Geometry check sheet. Reference: the model listing, model coordinates, mm. A direction names the side the tool comes from. Give positions to 0.01 mm unless a question says otherwise; leave off trailing zeros. Write each loop counter-clockwise with the first axis right and the second up, starting at its lowest first coordinate (ties: lowest second). Pieces come first, ordered by that corner, then holes. Notation, with made-up numbers: (36, 1.5) - (80, 1.5) arc R17 cw to (80, 13.5) - close; hole circle Ø6 at (-12.75, 73.5). An arc over 180 degrees is marked (long way). Write item = value, one per line. Start each with the question number.
(1) Depth check by flat-ended pin: pin 1 Ø1.5 at (x, y) = (-13, -8) entering from +Z; pin 2 Ø1.2 at (x, y) = (21, 17) entering from +Z; pin 3 Ø3 at (x, y) = (22.75, -17.5) entering from -Z. Enter the tip coordinate at first touch or a pass-through.
(2) Section check D-D, the plane y = 17.5. Enter the section's corners in (x, z).
(3) Section check A-A, the plane y = 0. Enter the section's corners in (x, z), plus the area to 3 significant figures.
(4) Section check B-B, the plane x = 16. Enter the section's corners in (y, z).
(5) Draft check along X on faces 4 (the flat face through (-23, -17, 6)), 5 (the flat face through (-21, -18, 1)), 6 (the flat face through (-24.2, 11.2, 18)), 7 (the flat face through (20, 17, 5)). Enter one of: pulls with the +X half, pulls with the -X half, needs draft (parallel to the pull), parting line crosses it, or undercut.
(6) Thickness scan on L1, parallel to Y at x = 22.75, z = 4.35; L2, parallel to X at y = -23, z = 17.25; L3, parallel to X at y = -17.5, z = 6.75. Record the ranges inside material, lowest first.
(7) Access from +Z, -Z, +X, -X, +Y, -Y to the whole of each face (thin tool, end or side, straight path). Record for faces 1 (the flat face through (-23, 18, 6)), 2 (the flat face through (-22, 18, 7)), 3 (the flat face through (-23, 15.5, 1)).
```python
from build123d import *

# Parameters (mm, degrees)
SKICA1_W                  = 50
SKICA1_H                  = 50
P_IDAT_VYSUNUT_M2_DEPTH   = 3
SKICA5_W                  = 50
SKICA5_H                  = 5
ODEBRAT_VYSUNUT_M3_DEPTH  = 1
P_IDAT_VYSUNUT_M9_DEPTH   = 15
SKICA17_R                 = 2
ODEBRAT_VYSUNUT_M8_DEPTH  = 4
SKICA18_W                 = 5
SKICA18_H                 = 5
P_IDAT_VYSUNUT_M10_DEPTH  = 7
SKICA19_W                 = 4
SKICA19_H                 = 4
ODEBRAT_VYSUNUT_M9_DEPTH  = 3
SKICA20_R                 = 1.25
ODEBRAT_VYSUNUT_M10_DEPTH = 3


with BuildPart() as part:
    # Skica1 → Přidat vysunutím2 (new body)
    with BuildSketch(Plane.XY):
        Rectangle(SKICA1_W, SKICA1_H)
    extrude(amount=P_IDAT_VYSUNUT_M2_DEPTH)

    # Skica5 → Odebrat vysunutím3 (cut)
    with BuildSketch(Plane(origin=(0, 0, 0), x_dir=(-1, 0, 0), z_dir=(0, 0, -1))):
        Rectangle(SKICA5_W, SKICA5_H)
    extrude(amount=-ODEBRAT_VYSUNUT_M3_DEPTH, mode=Mode.SUBTRACT)

    # Skica14 → Přidat vysunutím9 (add)
    with BuildSketch(Plane.XY.offset(3)):
        Polygon((25, 25), (-25, 25), (-25, -25), (-24, -25), (-24, 24), (24, 24), (24, -25), (25, -25), align=None)
    extrude(amount=P_IDAT_VYSUNUT_M9_DEPTH)

    # Skica17 → Odebrat vysunutím8 (cut)
    with BuildSketch(Plane(origin=(0, 0, 1), x_dir=(-1, 0, 0), z_dir=(0, 0, -1))):
        with Locations((-16, 0)):
            Circle(SKICA17_R)
        with Locations((16, 0)):
            Circle(SKICA17_R)
    extrude(amount=-ODEBRAT_VYSUNUT_M8_DEPTH, mode=Mode.SUBTRACT)

    # Skica18 → Přidat vysunutím10 (add)
    with BuildSketch(Plane(origin=(0, 0, 0), x_dir=(-1, 0, 0), z_dir=(0, 0, -1))):
        with Locations((-22.5, 17.5)):
            Rectangle(SKICA18_W, SKICA18_H)
        with Locations((-22.5, -17.5)):
            Rectangle(SKICA18_W, SKICA18_H)
        with Locations((22.5, -17.5)):
            Rectangle(SKICA18_W, SKICA18_H)
        with Locations((22.5, 17.5)):
            Rectangle(SKICA18_W, SKICA18_H)
    extrude(amount=-P_IDAT_VYSUNUT_M10_DEPTH)

    # Skica19 → Odebrat vysunutím9 (cut)
    with BuildSketch(Plane(origin=(0, 0, 0), x_dir=(-1, 0, 0), z_dir=(0, 0, -1))):
        with Locations((-23, 17.5)):
            Rectangle(SKICA19_W, SKICA19_H)
        with Locations((-23, -17.5)):
            Rectangle(SKICA19_W, SKICA19_H)
        with Locations((23, -17.5)):
            Rectangle(SKICA19_W, SKICA19_H)
        with Locations((23, 17.5)):
            Rectangle(SKICA19_W, SKICA19_H)
    extrude(amount=-ODEBRAT_VYSUNUT_M9_DEPTH, mode=Mode.SUBTRACT)

    # Skica20 → Odebrat vysunutím10 (cut)
    with BuildSketch(Plane(origin=(0, 0, 3), x_dir=(-1, 0, 0), z_dir=(0, 0, -1))):
        with Locations((-22.75, 17.5)):
            Circle(SKICA20_R)
        with Locations((22.75, 17.5)):
            Circle(SKICA20_R)
        with Locations((22.75, -17.5)):
            Circle(SKICA20_R)
        with Locations((-22.75, -17.5)):
            Circle(SKICA20_R)
    extrude(amount=-ODEBRAT_VYSUNUT_M10_DEPTH, mode=Mode.SUBTRACT)


solid = part.part
```
Model answer:
q1.pin_1 = 3
q1.pin_2 = 7
q1.pin_3 = 3
q2.outline = (-25, 3) - (-24, 3) - (-24, 6) - (-21.5, 6) - (-21.5, 3) - (-21, 3) - (-21, 0) - (21, 0) - (21, 3) - (21.5, 3) - (21.5, 6) - (24, 6) - (24, 3) - (25, 3) - (25, 18) - (24, 18) - (24, 7) - (20, 7) - (20, 3) - (-20, 3) - (-20, 7) - (-24, 7) - (-24, 18) - (-25, 18) - close
q3.outline = (-25, 1) - (-18, 1) - (-18, 3) - (-24, 3) - (-24, 18) - (-25, 18) - close; (-14, 1) - (14, 1) - (14, 3) - (-14, 3) - close; (18, 1) - (25, 1) - (25, 18) - (24, 18) - (24, 3) - (18, 3) - close
q3.area = 114 mm²
q4.outline = (-25, 0) - (-2.5, 0) - (-2.5, 1) - (-2, 1) - (-2, 3) - (-25, 3) - close; (2, 1) - (2.5, 1) - (2.5, 0) - (25, 0) - (25, 18) - (24, 18) - (24, 3) - (2, 3) - close
q5.face_4 = undercut
q5.face_5 = pulls with the -X half
q5.face_6 = needs draft
q5.face_7 = undercut
q6.L1 = -20 to -18.75, -16.25 to -15, 15 to 16.25, 18.75 to 20, 24 to 25
q6.L2 = -25 to -24, 24 to 25
q6.L3 = -25 to -20, 20 to 25
q7.face_1 = -Z
q7.face_2 = +Z, -Y
q7.face_3 = -Z, -X
